For this review, take the finished solid that the model builds, in its own axes (mm). Face numbers are marked on the shaded views. A direction names the side the tool comes from. Give positions to 0.01 mm unless a question says otherwise; leave off trailing zeros. Loops run counter-clockwise (first coordinate to the right, second up) from the corner with the lowest first, then second, coordinate; pieces in that order, holes last.
```python
from build123d import *

# Parameters (mm, degrees)
SKETCH_2_R          = 17.5
SKETCH_2_R_2        = 1.75
EXTRUDE_2_DEPTH     = 3
SKETCH_4_W          = 4.5
SKETCH_4_H          = 70
EXTRUDE_3_DEPTH     = 67
CUT_EXTRUDE_4_DEPTH = 71
SKETCH_6_R          = 2.25
SKETCH_6_W          = 21
SKETCH_6_H          = 41
CUT_EXTRUDE_6_DEPTH = 71
CUT_EXTRUDE_7_REACH = 72
SKETCH_7_R          = 1.75
SKETCH_8_R          = 4.5
CUT_EXTRUDE_8_DEPTH = 71
SKETCH_9_R          = 2.2
CUT_EXTRUDE_9_DEPTH = 4


with BuildPart() as part:
    # 草图2 → 凸台-拉伸2 (new body)
    with BuildSketch(Plane.XY):
        with BuildLine():
            Line((-31, -34), (-20.725119278, -34))
            Line((-20.725119278, -34), (-20.725119278, -38))
            ThreePointArc((-20.725119278, -38), (-19.553546403, -40.828427125), (-16.725119278, -42))
            Line((-16.725119278, -42), (16.725119278, -42))
            ThreePointArc((16.725119278, -42), (19.553546403, -40.828427125), (20.725119278, -38))
            Line((20.725119278, -38), (20.725119278, -34))
            Line((20.725119278, -34), (31, -34))
            ThreePointArc((31, -34), (33.828427125, -32.828427125), (35, -30))
            Line((35, -30), (35, 31))
            ThreePointArc((35, 31), (32.656854249, 36.656854249), (27, 39))
            Line((27, 39), (-27, 39))
            ThreePointArc((-27, 39), (-32.656854249, 36.656854249), (-35, 31))
            Line((-35, 31), (-35, -30))
            ThreePointArc((-35, -30), (-33.828427125, -32.828427125), (-31, -34))
        make_face()
        Circle(SKETCH_2_R, mode=Mode.SUBTRACT)
        with Locations((-17.324116139, 17.324116139)):
            Circle(SKETCH_2_R_2, mode=Mode.SUBTRACT)
        with Locations((17.324116139, 17.324116139)):
            Circle(SKETCH_2_R_2, mode=Mode.SUBTRACT)
        with Locations((17.324116139, -17.324116139)):
            Circle(SKETCH_2_R_2, mode=Mode.SUBTRACT)
        with Locations((-17.324116139, -17.324116139)):
            Circle(SKETCH_2_R_2, mode=Mode.SUBTRACT)
    extrude(amount=EXTRUDE_2_DEPTH)

    # 草图4 → 凸台-拉伸3 (add)
    with BuildSketch(Plane.XY.offset(3)):
        with Locations((32.75, -4)):
            Rectangle(SKETCH_4_W, SKETCH_4_H)
    extrude_3 = extrude(amount=EXTRUDE_3_DEPTH)

    # 草图5 → 切除-拉伸4 (cut, through all)
    with BuildSketch(Plane(origin=(35, 0, 0), x_dir=(0, 0, -1), z_dir=(1, 0, 0))):
        with BuildLine():
            ThreePointArc((-70, 21), (-67.071067812, 28.071067812), (-60, 31))
            Line((-60, 31), (-70, 31))
            Line((-70, 31), (-70, 21))
        make_face()
        with BuildLine():
            Line((-63.851082976, -30.192562933), (-70, 21))
            Line((-70, 21), (-70, -39))
            Line((-70, -39), (-53.922447942, -39))
            ThreePointArc((-53.922447942, -39), (-60.558499881, -36.480829811), (-63.851082976, -30.192562933))
        make_face()
        with BuildLine():
            Line((-3, -39), (-3, -30))
            Line((-3, -30), (-15.989445023, -37.624176182))
            ThreePointArc((-15.989445023, -37.624176182), (-18.428611976, -38.649916109), (-21.051419458, -39))
            Line((-21.051419458, -39), (-3, -39))
        make_face()
    cut_extrude_4 = extrude(amount=-CUT_EXTRUDE_4_DEPTH, mode=Mode.SUBTRACT)

    # 镜向2: 凸台-拉伸3, 切除-拉伸4 across plane
    add(extrude_3.mirror(Plane(origin=(0, 0, 0), x_dir=(0, 0, 1), z_dir=(1, 0, 0))))
    add(cut_extrude_4.mirror(Plane(origin=(0, 0, 0), x_dir=(0, 0, 1), z_dir=(1, 0, 0))), mode=Mode.SUBTRACT)

    # 草图6 → 切除-拉伸6 (cut, through all)
    with BuildSketch(Plane(origin=(35, 0, 0), x_dir=(0, 0, -1), z_dir=(1, 0, 0))):
        with Locations((-40, -29.315)):
            Circle(SKETCH_6_R)
        with Locations((-30, -29.315)):
            Circle(SKETCH_6_R)
        with Locations((-35, -5)):
            Rectangle(SKETCH_6_W, SKETCH_6_H)
        with Locations((-40, 19.315)):
            Circle(SKETCH_6_R)
        with Locations((-30, 19.315)):
            Circle(SKETCH_6_R)
    extrude(amount=-CUT_EXTRUDE_6_DEPTH, mode=Mode.SUBTRACT)

    # 草图7 → 切除-拉伸7 (cut, up to next)
    with BuildSketch(Plane(origin=(35, 0, 0), x_dir=(0, 0, -1), z_dir=(1, 0, 0)), mode=Mode.PRIVATE) as cut_extrude_7_sk1:
        with Locations((-60.5, 20.5)):
            Circle(SKETCH_7_R)
    cut_extrude_7_tool1 = extrude(cut_extrude_7_sk1.sketch, amount=-CUT_EXTRUDE_7_REACH, mode=Mode.PRIVATE) & part.part
    add(cut_extrude_7_tool1.solids().sort_by_distance((35, 20.5, 60.5))[0], mode=Mode.SUBTRACT)

    # 草图8 → 切除-拉伸8 (cut, through all)
    with BuildSketch(Plane(origin=(35, 0, 0), x_dir=(0, 0, -1), z_dir=(1, 0, 0))):
        with Locations((-16.97928935, -27)):
            Circle(SKETCH_8_R)
    extrude(amount=-CUT_EXTRUDE_8_DEPTH, mode=Mode.SUBTRACT)

    # 草图9 → 切除-拉伸9 (cut, through all)
    with BuildSketch(Plane.XY.offset(3)):
        with Locations((9, 28.65)):
            Circle(SKETCH_9_R)
        with Locations((-9, 28.65)):
            Circle(SKETCH_9_R)
        with Locations((5, -34.165)):
            Circle(SKETCH_9_R)
        with Locations((-5, -34.165)):
            Circle(SKETCH_9_R)
    extrude(amount=-CUT_EXTRUDE_9_DEPTH, mode=Mode.SUBTRACT)


solid = part.part
```
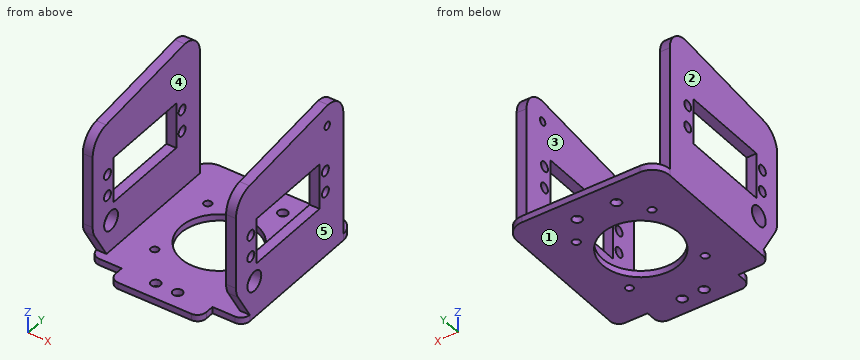
Item 1: Take a section at D-D on y = 12. Give the boundary of the cut face in (x, z), and give its area (3 significant figures).
Answer:
outline: (-35, 0) - (-12.74, 0) - (-12.74, 3) - (-30.5, 3) - (-30.5, 24.5) - (-35, 24.5) - close; (-35, 45.5) - (-30.5, 45.5) - (-30.5, 68.92) - (-35, 68.92) - close; (12.74, 0) - (35, 0) - (35, 24.5) - (30.5, 24.5) - (30.5, 3) - (12.74, 3) - close; (30.5, 45.5) - (35, 45.5) - (35, 68.92) - (30.5, 68.92) - close
area: 538 mm2
Item 2: For L1, parallel to Y at x = 31.9, z = 40 (3 decimals); L2, parallel to X at y = 16, z = 4; L3, parallel to Z at x = 16.5, y = 31, list the stretches that pass through material, from the lowest coordinate up.
Answer:
L1: y = -39 to -31.565, -27.065 to -25.5, 15.5 to 17.065, 21.565 to 31
L2: x = -35 to -30.5, 30.5 to 35
L3: z = 0 to 3
Item 3: Take a section at A-A on z = 50. Give the boundary of the cut face in (x, y), and give its area (3 significant figures).
Answer:
outline: (-35, -39) - (-30.5, -39) - (-30.5, 31) - (-35, 31) - close; (30.5, -39) - (35, -39) - (35, 31) - (30.5, 31) - close
area: 630 mm2
Item 4: The part is to be moulded in two halves that separate along X. For the marked faces 1, 2 and 3, say which applies: released by +X, released by -X, zero draft, split by the parting line, or undercut.
Answer:
face 1: zero draft
face 2: released by -X
face 3: undercut
Item 5: Take a section at B-B on z = 33.5. Give the boundary of the cut face in (x, y).
Answer:
outline: (-35, -39) - (-30.5, -39) - (-30.5, -25.5) - (-35, -25.5) - close; (-35, 15.5) - (-30.5, 15.5) - (-30.5, 31) - (-35, 31) - close; (30.5, -39) - (35, -39) - (35, -25.5) - (30.5, -25.5) - close; (30.5, 15.5) - (35, 15.5) - (35, 31) - (30.5, 31) - close
Item 6: Clearance check with flat-ended pins moving along their axes: pin 1 Ø4 at (x, y) = (-17.32, 17.32) entering from +Z; pin 2 Ø0.9 at (x, z) = (-25, 1.5) entering from -Y; pin 3 Ø1.3 at (x, y) = (-33.5, -1.5) entering from +Z. State where each tip first meets the part, or that it passes through.
Answer:
pin 1: stops at z = 3
pin 2: stops at y = -34
pin 3: stops at z = 67.38
Item 7: Tool access review of the marked faces 4 and 5: name each direction out of +Z, -Z, +X, -X, +Y, -Y from which nothing blocks a thin tool from reaching the whole face with its end or side.
Answer:
face 4: +Z, +Y, -Y
face 5: +Z, -Z, +X, +Y, -Y
Item 8: Take a section at C-C on x = -1. Give the boundary of the cut face in (y, z), and give its area (3 significant figures).
Answer:
outline: (-42, 0) - (-17.47, 0) - (-17.47, 3) - (-42, 3) - close; (17.47, 0) - (39, 0) - (39, 3) - (17.47, 3) - close
area: 138 mm2
